Geometry: see drawing. Coordinates: mm, zero at the bounding-box minimum. Coordinates: 2 decimals unless noted, no trailing zeros. Loops run counter-clockwise (first coordinate to the right, second up) from the corner with the lowest first, then second, coordinate; pieces in that order, holes last. Notation, with made-up numbers: (58, -9.5) - (84, -9.5) arc R24 ccw to (84, 17.5) - close; hole circle Ø1 at (69.25, 36.25). An arc over 180 degrees is marked (long way). Use a Markdown table: item, result. Add a question column.
1. Section query D-D on x = 36. Return the cut outline in (y, z).
2. Ray query, L1, parallel to X at y = 1.5, z = 2.75; L2, parallel to Y at x = 72, z = 1.2; L3, parallel to X at y = 7.5, z = 2.7. Return the intervals inside material, ascending. Write a range as [from, to].
3. Section query B-B on x = 72. Return the cut outline in (y, z), then the cut area to 3 significant figures.
4. Section query A-A on y = 18. Return the cut outline in (x, z), then the cut area to 3 significant figures.
5. Contact query for flat-ended pins moving along their axis: P1, Ø0.9, axis at y = 6.5, z = 2, coming from the -X side; P2, Ø0.9, axis at y = 2, z = 2, coming from the -X side; P3, Ø0.9, axis at y = 22.5, z = 1.5, coming from the +X side. Output: stop coordinate, or through.
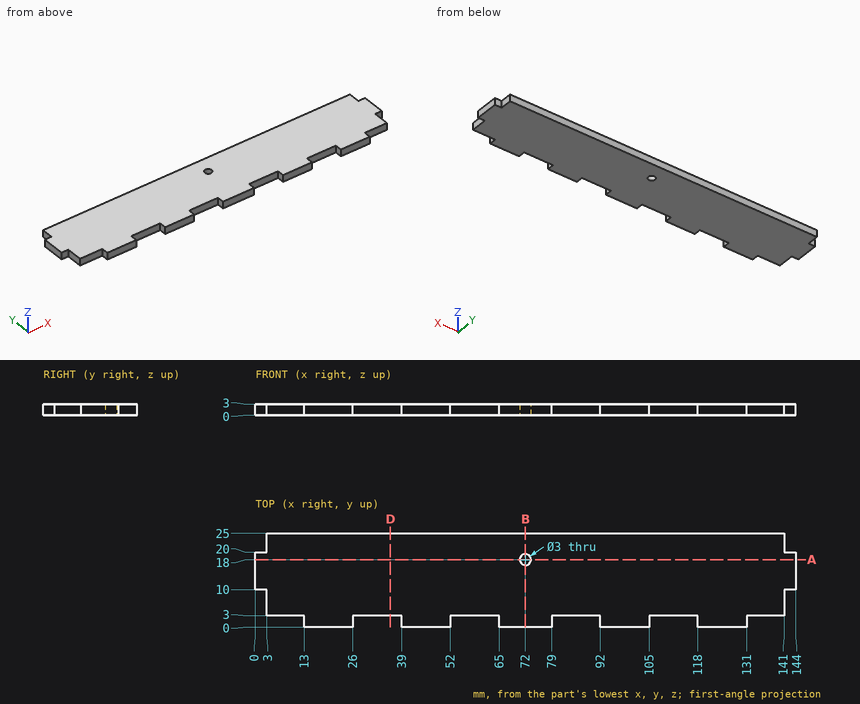
Resolved:
| question | item | result |
|---|---|---|
| 1 | outline | (3, 0) - (25, 0) - (25, 3) - (3, 3) - close |
| 2 | L1 | [13, 26], [39, 52], [65, 79], [92, 105], [118, 131] |
| 2 | L2 | [0, 16.5], [19.5, 25] |
| 2 | L3 | [3, 141] |
| 3 | outline | (0, 0) - (16.5, 0) - (16.5, 3) - (0, 3) - close; (19.5, 0) - (25, 0) - (25, 3) - (19.5, 3) - close |
| 3 | area | 66.0 mm² |
| 4 | outline | (0, 0) - (70.5, 0) - (70.5, 3) - (0, 3) - close; (73.5, 0) - (144, 0) - (144, 3) - (73.5, 3) - close |
| 4 | area | 423 mm² |
| 5 | P1 | x = 3 |
| 5 | P2 | x = 13 |
| 5 | P3 | x = 141 |
